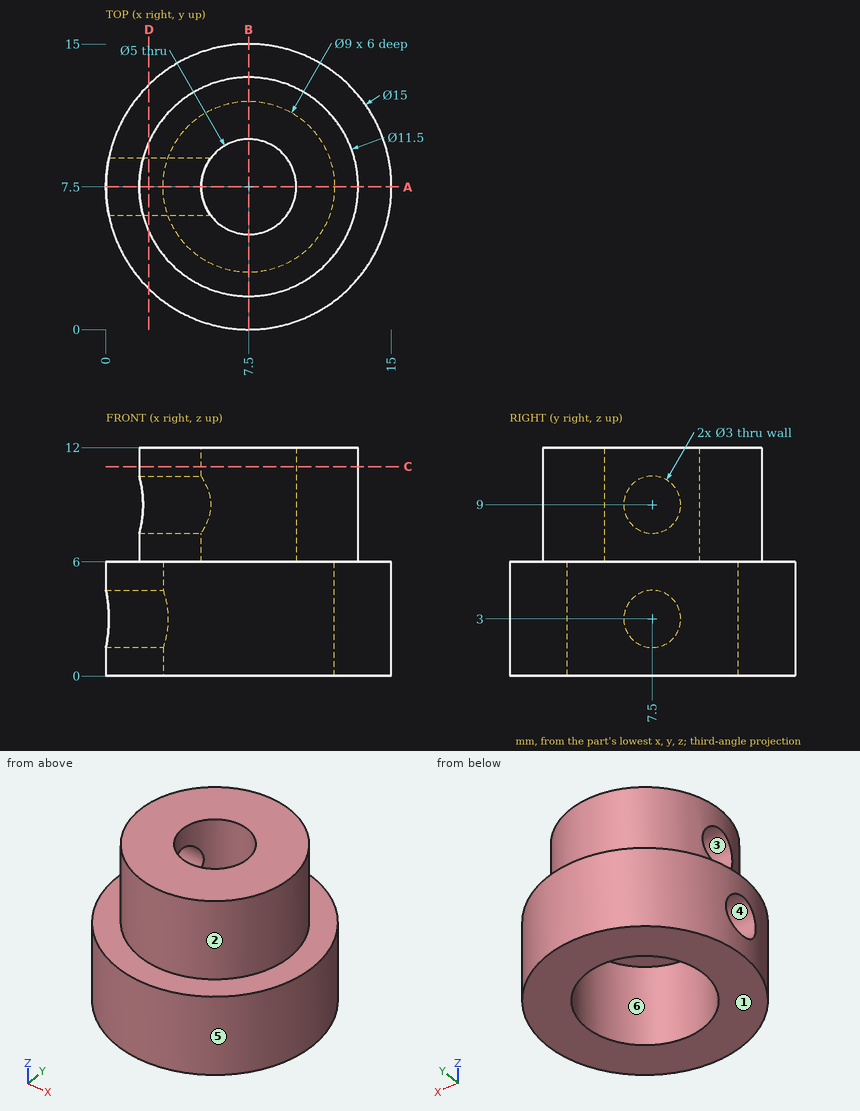
Study the drawing (mm; zero at the part's minimum x, y, z) and answer. A direction names the side the tool comes from. Give positions to 0.01 mm unless a question says otherwise; leave off trailing zeros. Loops run counter-clockwise (first coordinate to the right, second up) from the corner with the lowest first, then second, coordinate; pieces in that order, holes last. Notation, with made-up numbers: (-6.5, 64.5) -> (35.5, 64.5) arc R9 cw to (35.5, 81.5) -> close; hole circle Ø2 at (30, -4). An arc over 180 degrees is marked (long way). Use a Markdown table: item, result. Add a question column.
1) The part is cut by section B-B, the plane x = 7.5. Determine the outline of the cut face in (y, z).
2) The part is cut by section C-C, the plane z = 11. Determine the outline of the cut face in (x, y), plus the area to 3 significant figures.
3) The part is cut by section D-D, the plane x = 2.25. Determine the outline of the cut face in (y, z), plus the area to 3 significant figures.
4) Which of the six approach directions +Z, -Z, +X, -X, +Y, -Y give full straight-line access (tool end or side, diameter ignored) to the marked faces 1, 2 and 3?
5) Consider line 1 along Y through (x, z) = (7.5, 4); line 2 along Z through (x, y) = (11.5, 6.75); line 3 along Y through (x, z) = (10.5, 1.75). Determine where each line is inside the solid, lowest interval first.
6) The part is cut by section A-A, the plane y = 7.5. Determine the outline of the cut face in (x, z).
7) For a pull along X with two mould halves and no side action, classify the marked faces 4, 5 and 6 as +X half, -X half, draft (parallel to the pull), parting line (faces both ways), or undercut.
8) Each of these flat-tipped pins is pushed along its axis until it touches: P1, Ø3.5, axis at y = 7.5, z = 9, coming from the +X side; P2, Ø1.5, axis at x = 9, z = 7.5, coming from the -Y side; P3, Ø6.5, axis at x = 7.5, y = 7.5, coming from the -Z side. Where does it stop, or does it pass through?
Reported:
| question | item | result |
|---|---|---|
| 1 | outline | (0, 0) -> (3, 0) -> (3, 6) -> (5, 6) -> (5, 12) -> (1.75, 12) -> (1.75, 6) -> (0, 6) -> close; (10, 6) -> (12, 6) -> (12, 0) -> (15, 0) -> (15, 6) -> (13.25, 6) -> (13.25, 12) -> (10, 12) -> close |
| 2 | outline | circle Ø11.5 at (7.5, 7.5); hole circle Ø5 at (7.5, 7.5) |
| 2 | area | 84.2 mm^2 |
| 3 | outline | (2.14, 0) -> (12.86, 0) -> (12.86, 6) -> (9.85, 6) -> (9.85, 12) -> (5.15, 12) -> (5.15, 6) -> (2.14, 6) -> close; hole circle Ø3 at (7.5, 3); hole circle Ø3 at (7.5, 9) |
| 3 | area | 78.3 mm^2 |
| 4 | face 1 | -Z, +X, -X, +Y, -Y |
| 4 | face 2 | +Z |
| 4 | face 3 | -X |
| 5 | line 1 | y = 0 to 3, 12 to 15 |
| 5 | line 2 | z = 6 to 12 |
| 5 | line 3 | y = 0.63 to 4.15, 10.85 to 14.37 |
| 6 | outline | (0, 0) -> (3, 0) -> (3, 1.5) -> (0, 1.5) -> close; (0, 4.5) -> (3, 4.5) -> (3, 6) -> (5, 6) -> (5, 7.5) -> (1.75, 7.5) -> (1.75, 6) -> (0, 6) -> close; (1.75, 10.5) -> (5, 10.5) -> (5, 12) -> (1.75, 12) -> close; (10, 6) -> (12, 6) -> (12, 0) -> (15, 0) -> (15, 6) -> (13.25, 6) -> (13.25, 12) -> (10, 12) -> close |
| 7 | face 4 | draft |
| 7 | face 5 | parting line |
| 7 | face 6 | undercut |
| 8 | P1 | stops at x = 13.25 |
| 8 | P2 | stops at y = 1.8 |
| 8 | P3 | stops at z = 6 |
